```python
from build123d import *

# Parameters (mm, degrees)
BOSS_EXTRUDE1_DEPTH = 23
SKETCH2_R           = 8
CUT_EXTRUDE1_DEPTH  = 133.250640603
SKETCH3_R           = 18
SKETCH3_R_2         = 10
BOSS_EXTRUDE2_DEPTH = 5
CUT_EXTRUDE2_REACH  = 117.078
SKETCH4_R           = 10
BOSS_EXTRUDE3_REACH = 134.251
SKETCH5_R           = 6
CUT_EXTRUDE4_REACH  = 119.905
SKETCH7_R           = 6


with BuildPart() as part:
    # Sketch1 → Boss-Extrude1 (new, symmetric)
    with BuildSketch(Plane.XY):
        with BuildLine():
            Line((0, 0), (13, 0))
            Line((13, 0), (13, -20))
            ThreePointArc((13, -20), (15.369109272, -28.090772486), (21.728079924, -33.625821757))
            Line((21.728079924, -33.625821757), (32.590640025, -38.625821757))
            ThreePointArc((32.590640025, -38.625821757), (34.710296909, -40.470838181), (35.5, -43.167762343))
            Line((35.5, -43.167762343), (35.5, -93.167762343))
            Line((35.5, -93.167762343), (45.5, -93.167762343))
            Line((45.5, -93.167762343), (45.5, -43.167762343))
            ThreePointArc((45.5, -43.167762343), (43.130890728, -35.076989856), (36.771920076, -29.541940586))
            Line((36.771920076, -29.541940586), (25.909359975, -24.541940586))
            ThreePointArc((25.909359975, -24.541940586), (23.789703091, -22.696924162), (23, -20))
            Line((23, -20), (23, 6))
            ThreePointArc((23, 6), (21.828427125, 8.828427125), (19, 10))
            Line((19, 10), (-19, 10))
            ThreePointArc((-19, 10), (-21.828427125, 8.828427125), (-23, 6))
            Line((-23, 6), (-23, -20))
            ThreePointArc((-23, -20), (-23.789703091, -22.696924162), (-25.909359975, -24.541940586))
            Line((-25.909359975, -24.541940586), (-36.771920076, -29.541940586))
            ThreePointArc((-36.771920076, -29.541940586), (-43.130890728, -35.076989856), (-45.5, -43.167762343))
            Line((-45.5, -43.167762343), (-45.5, -93.167762343))
            Line((-45.5, -93.167762343), (-35.5, -93.167762343))
            Line((-35.5, -93.167762343), (-35.5, -43.167762343))
            ThreePointArc((-35.5, -43.167762343), (-34.710296909, -40.470838181), (-32.590640025, -38.625821757))
            Line((-32.590640025, -38.625821757), (-21.728079924, -33.625821757))
            ThreePointArc((-21.728079924, -33.625821757), (-15.369109272, -28.090772486), (-13, -20))
            Line((-13, -20), (-13, 0))
            Line((-13, 0), (0, 0))
        make_face()
    extrude(amount=BOSS_EXTRUDE1_DEPTH, both=True)

    # Sketch2 → Cut-Extrude1 (cut, through all)
    with BuildSketch(Plane(origin=(45.5, 0, 0), x_dir=(0, 0, -1), z_dir=(1, 0, 0))):
        with Locations(Location((0, -70.167762343, 0), (0, 0, 90))):
            Circle(SKETCH2_R)
        with BuildLine():
            ThreePointArc((0, -93.167762343), (-16.263455967, -86.43121831), (-23, -70.167762343))
            Line((-23, -70.167762343), (-23, -93.167762343))
            Line((-23, -93.167762343), (0, -93.167762343))
        make_face()
        with BuildLine():
            ThreePointArc((23, -70.167762343), (16.263455967, -86.43121831), (0, -93.167762343))
            Line((0, -93.167762343), (23, -93.167762343))
            Line((23, -93.167762343), (23, -70.167762343))
        make_face()
    extrude(amount=-CUT_EXTRUDE1_DEPTH, mode=Mode.SUBTRACT)

    # Sketch3 → Boss-Extrude2 (add)
    with BuildSketch(Plane(origin=(0, 10, 0), x_dir=(1, 0, 0), z_dir=(0, 1, 0))):
        with Locations(Location((0, 0, 0), (0, 0, 90))):
            Circle(SKETCH3_R)
        with Locations(Location((0, 0, 0), (0, 0, 270))):
            Circle(SKETCH3_R_2, mode=Mode.SUBTRACT)
    extrude(amount=BOSS_EXTRUDE2_DEPTH)

    # Sketch4 → Cut-Extrude2 (cut, up to next)
    with BuildSketch(Plane(origin=(0, 10, 0), x_dir=(1, 0, 0), z_dir=(0, 1, 0)), mode=Mode.PRIVATE) as cut_extrude2_sk1:
        with Locations(Location((0, 0, 0), (0, 0, 270))):
            Circle(SKETCH4_R)
    cut_extrude2_tool1 = extrude(cut_extrude2_sk1.sketch, amount=-CUT_EXTRUDE2_REACH, mode=Mode.PRIVATE) & part.part
    add(cut_extrude2_tool1.solids().sort_by_distance((0, 10, 0))[0], mode=Mode.SUBTRACT)

    # Sketch5 → Boss-Extrude3 (add, up to next)
    with BuildSketch(Plane(origin=(45.5, 0, 0), x_dir=(0, 0, -1), z_dir=(1, 0, 0)), mode=Mode.PRIVATE) as boss_extrude3_sk1:
        with BuildLine():
            Line((5, -60.379262018), (5, -19))
            ThreePointArc((5, -19), (0, 6), (-5, -19))
            Line((-5, -19), (-5, -60.379262018))
            Line((-5, -60.379262018), (5, -60.379262018))
        make_face()
        with Locations(Location((0, -7, 0), (0, 0, 90))):
            Circle(SKETCH5_R, mode=Mode.SUBTRACT)
    boss_extrude3_tool1 = extrude(boss_extrude3_sk1.sketch, amount=-BOSS_EXTRUDE3_REACH, mode=Mode.PRIVATE) - part.part
    boss_extrude3 = boss_extrude3_tool1.solids().sort_by_distance((45.5, -23.296906, 0))[0]
    add(boss_extrude3)

    # Sketch7 → Cut-Extrude4 (cut, up to next)
    with BuildSketch(Plane(origin=(23, 0, 0), x_dir=(0, 0, -1), z_dir=(1, 0, 0)), mode=Mode.PRIVATE) as cut_extrude4_sk1:
        with Locations(Location((0, -7, 0), (0, 0, 90))):
            Circle(SKETCH7_R)
    cut_extrude4_tool1 = extrude(cut_extrude4_sk1.sketch, amount=-CUT_EXTRUDE4_REACH, mode=Mode.PRIVATE) & part.part
    cut_extrude4 = cut_extrude4_tool1.solids().sort_by_distance((23, -7, 0))[0]
    add(cut_extrude4, mode=Mode.SUBTRACT)

    # Mirror1: Boss-Extrude3, Cut-Extrude4 across plane
    add(boss_extrude3.mirror(Plane(origin=(0, 0, 0), x_dir=(0, 0, 1), z_dir=(1, 0, 0))))
    add(cut_extrude4.mirror(Plane(origin=(0, 0, 0), x_dir=(0, 0, 1), z_dir=(1, 0, 0))), mode=Mode.SUBTRACT)


solid = part.part
```
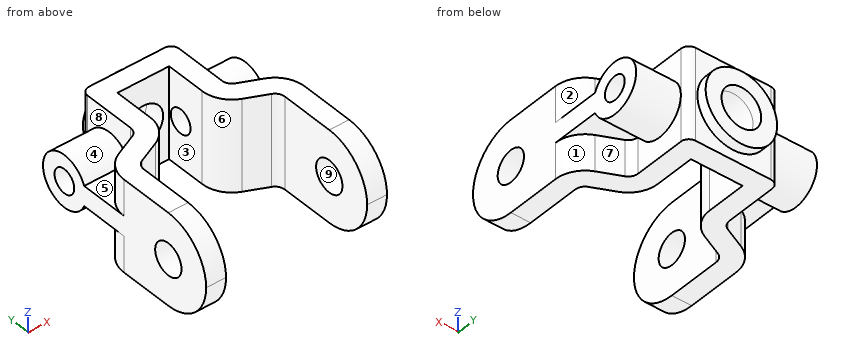
For this review, take the finished solid that the model builds, in its own axes (mm). Face numbers are marked on the shaded views. A direction names the side the tool comes from. Round coordinates to 2 decimals unless told otherwise and drop trailing zeros. Write each loop counter-clockwise with the first axis right and the second up, starting at its lowest first coordinate (ties: lowest second). Pieces come first, ordered by that corner, then holes. Notation, with made-up numbers: (32.25, 54.5) - (89.25, 54.5) arc R33 ccw to (89.25, 83.5) - close; hole circle Ø2 at (62.5, 36). An arc over 180 degrees is marked (long way). Write each question's results on one line, items separated by ' | '.
Item 1: Take a section at D-D on x = -34. State the section outline as (y, z) points, then the cut area to 4 significant figures.
Calculated:
outline: (-39.6, -23) - (-28.27, -23) - (-28.27, -5) - (-19, -5) arc R13 ccw (long way) to (-19, 5) - (-28.27, 5) - (-28.27, 23) - (-39.6, 23) - close; hole circle Ø12 at (-7, 0) | area: 1,025 mm^2
Item 2: For pin 1 (3 mm diameter, centred on x = -20, z = 13, fed in from -Y); pin 2 (4 mm diameter, centred on x = 18.5, z = 8.5, fed in from +Y), all flat-tipped, find the tip position at first contact; note any pin that passes through.
Calculated:
pin 1: stops at y = -33.52 | pin 2: stops at y = 10
Item 3: For the marked faces 1, 2, 3, 4 and 5, list the 3-axis set-ups (+Z, -Z, +X, -X, +Y, -Y) from which the entire face can be reached by the end or side of a thin tool; tool diameter is ignored.
Calculated:
face 1: -Z, +X | face 2: +Z, +X | face 3: +Z, -Z, -Y | face 4: -X | face 5: +Z, -X
Item 4: Draft analysis for pull direction X (two halves, no side actions). For the marked faces 6, 7, 8 and 9, state which applies: pulls with the +X half, pulls with the -X half, needs draft (parallel to the pull), parting line crosses it, or undercut.
Calculated:
face 6: undercut | face 7: pulls with the +X half | face 8: pulls with the -X half | face 9: needs draft
Item 5: Take a section at B-B on y = -7. State the section outline as (x, z) points.
Calculated:
outline: (-45.5, -13) - (-23, -13) - (-23, -23) - (-13, -23) - (-13, -6) - (-45.5, -6) - close; (-45.5, 6) - (-13, 6) - (-13, 23) - (-23, 23) - (-23, 13) - (-45.5, 13) - close; (13, -23) - (23, -23) - (23, -13) - (45.5, -13) - (45.5, -6) - (13, -6) - close; (13, 6) - (45.5, 6) - (45.5, 13) - (23, 13) - (23, 23) - (13, 23) - close
Item 6: Take a section at A-A on x = 0. State the section outline as (y, z) points, then the cut area to 3 significant figures.
Calculated:
outline: (0, -23) - (10, -23) - (10, -18) - (15, -18) - (15, -10) - (0, -10) - close; (0, 10) - (15, 10) - (15, 18) - (10, 18) - (10, 23) - (0, 23) - close | area: 340 mm^2
Item 7: Take a section at C-C on y = -84.5. State the section outline as (x, z) points, then the cut area to 3 significant figures.
Calculated:
outline: (-45.5, -17.99) - (-35.5, -17.99) - (-35.5, 17.99) - (-45.5, 17.99) - close; (35.5, -17.99) - (45.5, -17.99) - (45.5, 17.99) - (35.5, 17.99) - close | area: 720 mm^2
Item 8: To check wall thickness, follow line 1 along Z through (x, y) = (38, -7); line 2 along X through (y, z) = (-58, 12); line 3 along X through (y, z) = (-13, 9). State the ranges of each line that lie inside material, in increasing order. Write a range as from..to.
Calculated:
line 1: z = -13..-6, 6..13 | line 2: x = -45.5..-35.5, 35.5..45.5 | line 3: x = -45.5..-13, 13..45.5
